Design review of the part built by this model. Coordinates are the model's own, in mm. A direction names the side the tool comes from. Give positions to 0.01 mm unless a question says otherwise; leave off trailing zeros. Loops run counter-clockwise (first coordinate to the right, second up) from the corner with the lowest first, then second, coordinate; pieces in that order, holes last. Notation, with made-up numbers: (75, 39) -> (129, 39) arc R26 ccw to (129, 74) -> close; hole circle Ø4 at (3.25, -4). An arc over 180 degrees is marked (long way). Use a Markdown table: item, result. Add a question column.
1. For faces 5 (the flat face through (0, -42, 0)), 6 (the flat face through (0, 40, 11)), list the 3-axis set-ups (+Z, -Z, +X, -X, +Y, -Y) from which the entire face can be reached by the end or side of a thin tool; tool diameter is ignored.
2. Add section B-B (y = 0). State the section outline as (x, z) points, and give its area (4 significant figures).
3. Add section D-D (x = -13). State the section outline as (y, z) points, and give its area (3 significant figures).
4. Draft analysis for pull direction X (two halves, no side actions). For faces 1 (the cylindrical face through (-6.38, -43.87, 5.42)), 2 (the flat face through (24, 14, 24)), 3 (the flat face through (0, -42, 11)), 4 (the cylindrical face through (-20.091, -52.293, 5.423)), state which applies: pulls with the +X half, pulls with the -X half, needs draft (parallel to the pull), parting line crosses it, or undercut.
5. To check wall thickness, follow line 1 (Y direction, x = -11, z = 4); line 2 (X direction, y = -40, z = 10); line 3 (Y direction, x = 14, z = 3). State the ranges of each line that lie inside material, in increasing order.
6. Add section A-A (z = 10). State the section outline as (x, y) points.
7. Add section C-C (z = 26). State the section outline as (x, y) points, and give its area (3 significant figures).
8. For pin 1 Ø3 at (x, y) = (0, 0) entering from -Z; pin 2 Ø16 at (x, y) = (11, -41.96) entering from +Z; pin 3 Ø4 at (x, y) = (5, 14) entering from +Z; pin 4 Ø24 at (x, y) = (-0.5, 34.5) entering from +Z, all flat-tipped, find the tip position at first contact; note any pin that passes through.
```python
from build123d import *

# Parameters (mm, degrees)
F1_DEPTH = 24
F2_R     = 2.5
F2_R_2   = 5
F3_DEPTH = 30.001
F4_R     = 13
F5_R     = 2


with BuildPart() as f1:
    # F0 (on Right) → F1 (new body, symmetric)
    with BuildSketch(Plane.YZ):
        with BuildLine():
            Line((-56, 0), (-30, 0))
            ThreePointArc((-30, 0), (-29.4730143031, 5.5983415304), (-27.9105714739, 11))
            Line((-27.9105714739, 11), (-56, 11))
            Line((-56, 11), (-56, 0))
        make_face()
        with BuildLine():
            Line((-30, 0), (-27.5, 0))
            ThreePointArc((-27.5, 0), (-26.9199236056, 5.6185152015), (-25.2041663223, 11))
            Line((-25.2041663223, 11), (-27.9105714739, 11))
            ThreePointArc((-27.9105714739, 11), (-29.4730143031, 5.5983415304), (-30, 0))
        make_face()
        with BuildLine():
            ThreePointArc((-25.2041663223, 11), (0, 27.5), (25.2041663223, 11))
            Line((25.2041663223, 11), (27.9105714739, 11))
            ThreePointArc((27.9105714739, 11), (0, 30), (-27.9105714739, 11))
            Line((-27.9105714739, 11), (-25.2041663223, 11))
        make_face()
        with BuildLine():
            ThreePointArc((25.2041663223, 11), (26.9199236056, 5.6185152015), (27.5, 0))
            Line((27.5, 0), (30, 0))
            ThreePointArc((30, 0), (29.4730143031, 5.5983415304), (27.9105714739, 11))
            Line((27.9105714739, 11), (25.2041663223, 11))
        make_face()
        with BuildLine():
            ThreePointArc((27.9105714739, 11), (29.4730143031, 5.5983415304), (30, 0))
            Line((30, 0), (51, 0))
            Line((51, 0), (51, 11))
            Line((51, 11), (40, 11))
            Line((40, 11), (27.9105714739, 11))
        make_face()
    extrude(amount=F1_DEPTH, both=True)

    # F2 (on Top) → F3 (cut, through all)
    with BuildSketch(Plane.XY):
        Circle(F2_R)
        with Locations((-11, -41.955285737)):
            Circle(F2_R_2)
        with Locations((11, -41.955285737)):
            Circle(F2_R_2)
    extrude(amount=F3_DEPTH, mode=Mode.SUBTRACT)

    # F4
    f4_edges = [f1.edges().sort_by_distance(p)[0] for p in [
        (24, -56, 5.5),
        (-24, -56, 5.5),
    ]]
    fillet(f4_edges, radius=F4_R)

    # F5
    f5_edges = [f1.edges().sort_by_distance(p)[0] for p in [
        (0, -27.910571, 11),
        (0, 27.910571, 11),
    ]]
    fillet(f5_edges, radius=F5_R)


solid = f1.part
```
Taken from the geometry:
| question | item | result |
|---|---|---|
| 1 | face 5 | -Z, +X, -X, +Y, -Y |
| 1 | face 6 | +Z, +X, -X, +Y |
| 2 | outline | (-24, 27.5) -> (-2.5, 27.5) -> (-2.5, 30) -> (-24, 30) -> close; (2.5, 27.5) -> (24, 27.5) -> (24, 30) -> (2.5, 30) -> close |
| 2 | area | 107.5 mm^2 |
| 3 | outline | (-55.85, 0) -> (-46.54, 0) -> (-46.54, 11) -> (-55.85, 11) -> close; (-37.37, 0) -> (-27.5, 0) arc R27.5 cw to (27.5, 0) -> (51, 0) -> (51, 11) -> (29.24, 11) arc R2 cw to (27.41, 12.19) arc R30 ccw to (-27.41, 12.19) arc R2 cw to (-29.24, 11) -> (-37.37, 11) -> close |
| 3 | area | 656 mm^2 |
| 4 | face 1 | undercut |
| 4 | face 2 | pulls with the +X half |
| 4 | face 3 | needs draft |
| 4 | face 4 | pulls with the -X half |
| 5 | line 1 | y = -56 to -46.96, -36.96 to -27.21, 27.21 to 51 |
| 5 | line 2 | x = -24 to -15.6, -6.4 to 6.4, 15.6 to 24 |
| 5 | line 3 | y = -55.65 to -45.96, -37.96 to -27.34, 27.34 to 51 |
| 6 | outline | (-24, -43) arc R13 ccw to (-11, -56) -> (11, -56) arc R13 ccw to (24, -43) -> (24, -25.62) -> (-24, -25.62) -> close; (-24, 25.62) -> (24, 25.62) -> (24, 51) -> (-24, 51) -> close; hole circle Ø10 at (-11, -41.96); hole circle Ø10 at (11, -41.96) |
| 7 | outline | (-24, -14.97) -> (24, -14.97) -> (24, -8.96) -> (-24, -8.96) -> close; (-24, 8.96) -> (24, 8.96) -> (24, 14.97) -> (-24, 14.97) -> close |
| 7 | area | 577 mm^2 |
| 8 | pin 1 | passes through |
| 8 | pin 2 | stops at z = 11 |
| 8 | pin 3 | stops at z = 27.5 |
| 8 | pin 4 | stops at z = 19.84 |
